from build123d import *

# Parameters (mm, degrees)
CROQUIS1_R              = 1.7
SALIENTE_EXTRUIR1_DEPTH = 2
CROQUIS2_R              = 2.55
CROQUIS2_R_2            = 1.7
SALIENTE_EXTRUIR2_DEPTH = 8


with BuildPart() as part:
    # Croquis1 → Saliente-Extruir1 (new body)
    with BuildSketch(Plane.XY):
        with BuildLine():
            ThreePointArc((-1.584158416, 1.972702708), (-5.75, 0), (-1.584158416, -1.972702708))
            ThreePointArc((-1.584158416, -1.972702708), (0, -1.406724971), (1.584158416, -1.972702708))
            ThreePointArc((1.584158416, -1.972702708), (5.75, 0), (1.584158416, 1.972702708))
            ThreePointArc((1.584158416, 1.972702708), (0, 1.406724971), (-1.584158416, 1.972702708))
        make_face()
        with Locations((-3.2, 0)):
            Circle(CROQUIS1_R, mode=Mode.SUBTRACT)
        with Locations(Location((3.2, 0, 0), (0, 0, 180))):
            Circle(CROQUIS1_R, mode=Mode.SUBTRACT)
    saliente_extruir1 = extrude(amount=SALIENTE_EXTRUIR1_DEPTH)

    # Croquis2 → Saliente-Extruir2 (add)
    # profile 1 of 2: a face of its own
    with BuildSketch(Plane.XY.offset(2)):
        with Locations(Location((-3.2, 0, 0), (0, 0, 309.320919198))):
            Circle(CROQUIS2_R)
        with Locations((-3.2, 0)):
            Circle(CROQUIS2_R_2, mode=Mode.SUBTRACT)
    # profile 2 of 2: a face of its own
    with BuildSketch(Plane.XY.offset(2)):
        with Locations(Location((3.2, 0, 0), (0, 0, 129.320919198))):
            Circle(CROQUIS2_R)
        with Locations(Location((3.2, 0, 0), (0, 0, 180))):
            Circle(CROQUIS2_R_2, mode=Mode.SUBTRACT)
    extrude(amount=SALIENTE_EXTRUIR2_DEPTH)

    # Simetría1: Saliente-Extruir1 across plane
    add(saliente_extruir1.mirror(Plane.XY.offset(6)))


solid = part.part
Geometry check sheet. Reference: the model listing, model coordinates, mm. A direction names the side the tool comes from. Coordinates: 2 decimals unless noted, no trailing zeros. Order: outer loops, then holes, each group sorted by start corner. A loop starts at its lowest first (then second) coordinate and runs counter-clockwise, first axis right, second up. Notation, with made-up numbers: (47.5, 81.5) - (58.5, 81.5) arc R27 ccw to (58.5, 97.5) - close; hole circle Ø7 at (28, -40). An arc over 180 degrees is marked (long way). One line per item, written item: value.
(1) Sectioned sample at C-C (x = -3.2). Enter the section's corners in (y, z), and give its area (3 significant figures).
Data:
outline: (-2.55, 0) - (-1.7, 0) - (-1.7, 12) - (-2.55, 12) - close; (1.7, 0) - (2.55, 0) - (2.55, 12) - (1.7, 12) - close
area: 20.4 mm^2
(2) Depth check by flat-ended pin: pin 1 Ø3 at (x, y) = (3.2, 0) entering from -Z; pin 2 Ø1 at (y, z) = (0.5, 3.5) entering from +X. Enter the tip coordinate at first touch or a pass-through.
Data:
pin 1: passes through
pin 2: stops at x = 5.75
(3) Thickness scan on probe 1 along Y at (x, z) = (-3.2, 5.75); probe 2 along X at (y, z) = (0.65, 9.75); probe 3 along X at (y, z) = (0.55, 11). Record the ranges inside material, lowest first. Write a range as from..to.
Data:
probe 1: y = -2.55..-1.7, 1.7..2.55
probe 2: x = -5.67..-4.77, -1.63..-0.73, 0.73..1.63, 4.77..5.67
probe 3: x = -5.69..-4.81, -1.59..1.59, 4.81..5.69
(4) Access from +Z, -Z, +X, -X, +Y, -Y to the whole of each face (thin tool, end or side, straight path). Record for faces 1 (the face through (0, 0, 2)), 2 (the face through (-0.024, -1.407, 11.014)).
Data:
face 1: none
face 2: +Z, -Z, -Y
(5) Sectioned sample at A-A (y = 0). Enter the section's corners in (x, z).
Data:
outline: (-5.75, 0) - (-4.9, 0) - (-4.9, 12) - (-5.75, 12) - close; (-1.5, 0) - (1.5, 0) - (1.5, 12) - (-1.5, 12) - close; (4.9, 0) - (5.75, 0) - (5.75, 12) - (4.9, 12) - close; hole (-0.65, 2) - (0.65, 2) - (0.65, 10) - (-0.65, 10) - close
(6) Sectioned sample at D-D (y = 2.25). Enter the section's corners in (x, z).
Data:
outline: (-4.4, 0) - (-2, 0) - (-2, 12) - (-4.4, 12) - close; (2, 0) - (4.4, 0) - (4.4, 12) - (2, 12) - close
(7) Sectioned sample at B-B (z = 8.75). Enter the section's corners in (x, y), and give its area (3 significant figures).
Data:
outline: circle Ø5.1 at (-3.2, 0); circle Ø5.1 at (3.2, 0); hole circle Ø3.4 at (-3.2, 0); hole circle Ø3.4 at (3.2, 0)
area: 22.7 mm^2
(8) Release check for a two-part mould opening along X. For faces 3 (the face through (0, 0, 10)), 4 (the face through (0, 0, 12)) record: +X half, -X half, draft (parallel to the pull), parting line (faces both ways), or undercut.
Data:
face 3: undercut
face 4: draft
